Input: part model. Units: mm. Frame: model coordinates. Face numbers are marked on the shaded views. A direction names the side the tool comes from. Coordinates: 2 decimals unless noted, no trailing zeros. Order: outer loops, then holes, each group sorted by start corner. A loop starts at its lowest first (then second) coordinate and runs counter-clockwise, first axis right, second up. Notation, with made-up numbers: M -27,5 L 13,5 A28 ccw 13,34 Z; hole C 21,28.5 d2. An arc over 180 degrees is marked long. One line per item, written item: value.
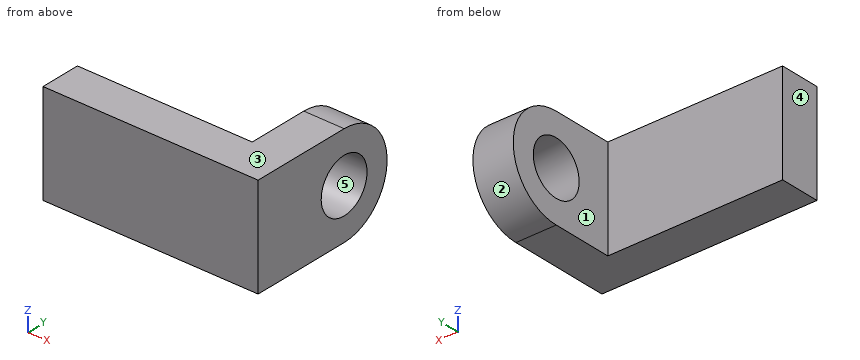
```python
from build123d import *

# Parameters (mm, degrees)
CROQUIS1_W              = 130
CROQUIS1_H              = 75
SALIENTE_EXTRUIR1_DEPTH = 30
SALIENTE_EXTRUIR2_DEPTH = 30
CROQUIS3_R              = 20
CORTAR_EXTRUIR1_DEPTH   = 62


with BuildPart() as part:
    # Croquis1 → Saliente-Extruir1 (new body)
    with BuildSketch(Plane(origin=(0, 0, 0), x_dir=(1, 0, 0), z_dir=(0, 1, 0))):
        Rectangle(CROQUIS1_W, CROQUIS1_H)
    extrude(amount=SALIENTE_EXTRUIR1_DEPTH)

    # Croquis2 → Saliente-Extruir2 (add)
    with BuildSketch(Plane(origin=(65, 0, 0), x_dir=(0, 0, -1), z_dir=(1, 0, 0))):
        with BuildLine():
            Line((-37.5, 0), (37.5, 0))
            Line((37.5, 0), (37.5, 75))
            ThreePointArc((37.5, 75), (0, 112.5), (-37.5, 75))
            Line((-37.5, 75), (-37.5, 0))
        make_face()
    extrude(amount=SALIENTE_EXTRUIR2_DEPTH)

    # Croquis3 → Cortar-Extruir1 (cut)
    with BuildSketch(Plane(origin=(95, 0, 0), x_dir=(0, 0, -1), z_dir=(1, 0, 0))):
        with Locations((0, 75)):
            Circle(CROQUIS3_R)
    extrude(amount=-CORTAR_EXTRUIR1_DEPTH, mode=Mode.SUBTRACT)


solid = part.part
```
(1) Access query for the marked faces 1 and 2. Directions: +Z, -Z, +X, -X, +Y, -Y. A direction counts if a zero-diameter tool reaches every point of the face in a straight line with its end or side. Return the directions, or none.
Data:
face 1: +Z, -Z, -X, +Y
face 2: +X, -X, +Y
(2) Cut plane B-B on z = -13.5. Output: boundary loops of the cut face in (x, y), plus the area to 3 significant figures.
Data:
outline: M -65,0 L 95,0 L 95,60.24 L 65,60.24 L 65,30 L -65,30 Z; M 65,89.76 L 95,89.76 L 95,109.99 L 65,109.99 Z
area: 6,310 mm2
(3) Ray query, line 1 (Y direction, x = 87, z = 0); line 2 (Y direction, x = -18.5, z = -25.5); line 3 (X direction, y = 99, z = 28). Return the intervals inside material, ascending. Write a range as from..to.
Data:
line 1: y = 0..55, 95..112.5
line 2: y = 0..30
line 3: x = 65..95
(4) Cut plane D-D on z = 0. Output: boundary loops of the cut face in (x, y), plus the area to 4 significant figures.
Data:
outline: M -65,0 L 95,0 L 95,55 L 65,55 L 65,30 L -65,30 Z; M 65,95 L 95,95 L 95,112.5 L 65,112.5 Z
area: 6,075 mm2
(5) Cut plane C-C on y = 58. Output: boundary loops of the cut face in (x, z).
Data:
outline: M 65,-37.5 L 95,-37.5 L 95,-10.54 L 65,-10.54 Z; M 65,10.54 L 95,10.54 L 95,37.5 L 65,37.5 Z
(6) Cut plane A-A on x = 76.5. Output: boundary loops of the cut face in (y, z), plus the area to 3 significant figures.
Data:
outline: M 0,-37.5 L 75,-37.5 A37.5 ccw 75,37.5 L 0,37.5 Z; hole C 75,0 d40
area: 6,580 mm2
(7) First-contact query: pin 1 (3 mm diameter, centred on x = 11.5, z = -29.5, fed in from +Y); pin 2 (22.5 mm diameter, centred on y = 65, z = -18, fed in from -X); pin 3 (1 mm diameter, centred on x = -44.5, z = 1, fed in from -Y). Flat tips, straight axial feed; report the tip coordinate or a pass-through.
Data:
pin 1: stops at y = 30
pin 2: stops at x = 65
pin 3: stops at y = 0
(8) Draft query along Z for the marked faces 3, 4 and 5. Return one class per face: released by +Z, released by -Z, zero draft, split by the parting line, or undercut.
Data:
face 3: released by +Z
face 4: zero draft
face 5: undercut
